```python
from build123d import *

# Parameters (mm, degrees)
STRUCTURAL_MEMBER1_DEPTH = 500
CUT_EXTRUDE1_REACH       = 252.724
LPATTERN1_COUNT          = 196
LPATTERN1_PITCH          = 24.892
SKETCH4_W                = 4000
SKETCH4_H                = 182.847095399
CUT_EXTRUDE2_DEPTH       = 140
SKETCH5_W                = 3.509513676
SKETCH5_H                = 55.564681105
CUT_EXTRUDE3_DEPTH       = 140


with BuildPart() as part:
    # Sketch2 → Structural Member1 (new body)
    with BuildSketch(Plane(origin=(-250, 0, 0), x_dir=(0, 0, -1), z_dir=(1, 0, 0))):
        with BuildLine():
            Line((0, 12.25), (0, -12.25))
            ThreePointArc((0, -12.25), (-0.366116524, -13.133883476), (-1.25, -13.5))
            Line((-1.25, -13.5), (-5.25, -13.5))
            ThreePointArc((-5.25, -13.5), (-6.133883476, -13.866116524), (-6.5, -14.75))
            Line((-6.5, -14.75), (-6.5, -17.5))
            Line((-6.5, -17.5), (-7.5, -17.5))
            Line((-7.5, -17.5), (-7.5, -14.75))
            ThreePointArc((-7.5, -14.75), (-6.840990258, -13.159009742), (-5.25, -12.5))
            Line((-5.25, -12.5), (-1.25, -12.5))
            ThreePointArc((-1.25, -12.5), (-1.073223305, -12.426776695), (-1, -12.25))
            Line((-1, -12.25), (-1, 12.25))
            ThreePointArc((-1, 12.25), (-1.073223305, 12.426776695), (-1.25, 12.5))
            Line((-1.25, 12.5), (-5.25, 12.5))
            ThreePointArc((-5.25, 12.5), (-6.840990258, 13.159009742), (-7.5, 14.75))
            Line((-7.5, 14.75), (-7.5, 17.5))
            Line((-7.5, 17.5), (-6.5, 17.5))
            Line((-6.5, 17.5), (-6.5, 14.75))
            ThreePointArc((-6.5, 14.75), (-6.133883476, 13.866116524), (-5.25, 13.5))
            Line((-5.25, 13.5), (-1.25, 13.5))
            ThreePointArc((-1.25, 13.5), (-0.366116524, 13.133883476), (0, 12.25))
        make_face()
    extrude(amount=STRUCTURAL_MEMBER1_DEPTH)

    # Sketch3 → Cut-Extrude1 (cut, up to next)
    with BuildSketch(Plane.XY, mode=Mode.PRIVATE) as cut_extrude1_sk1:
        with BuildLine():
            Line((-241.745, 3.175), (-230.315, 3.175))
            ThreePointArc((-230.315, 3.175), (-227.14, 0), (-230.315, -3.175))
            Line((-230.315, -3.175), (-241.745, -3.175))
            ThreePointArc((-241.745, -3.175), (-244.92, 0), (-241.745, 3.175))
        make_face()
    cut_extrude1_tool1 = extrude(cut_extrude1_sk1.sketch, amount=CUT_EXTRUDE1_REACH, mode=Mode.PRIVATE) & part.part
    cut_extrude1 = cut_extrude1_tool1.solids().sort_by_distance((-236.03, 0, 0))[0]
    add(cut_extrude1, mode=Mode.SUBTRACT)

    # LPattern1: Cut-Extrude1 ×196
    with Locations(*[(i * LPATTERN1_PITCH, 0, 0) for i in range(1, LPATTERN1_COUNT)]):
        add(cut_extrude1, mode=Mode.SUBTRACT)

    # Sketch4 → Cut-Extrude2 (cut)
    with BuildSketch(Plane.XY.offset(7.5)):
        with Locations((-1947.5, -12.909953422)):
            Rectangle(SKETCH4_W, SKETCH4_H)
    extrude(amount=-CUT_EXTRUDE2_DEPTH, mode=Mode.SUBTRACT)

    # Sketch5 → Cut-Extrude3 (cut)
    with BuildSketch(Plane.XY.offset(7.5)):
        with Locations((249.254756838, -3.17340083)):
            Rectangle(SKETCH5_W, SKETCH5_H)
    extrude(amount=-CUT_EXTRUDE3_DEPTH, mode=Mode.SUBTRACT)


solid = part.part
```
Design review of the part built by this model. Coordinates are the model's own, in mm. A direction names the side the tool comes from. Give positions to 0.01 mm unless a question says otherwise; leave off trailing zeros. Write each loop counter-clockwise with the first axis right and the second up, starting at its lowest first coordinate (ties: lowest second). Pieces come first, ordered by that corner, then holes. Notation, with made-up numbers: (-12, 65.5) - (8, 65.5) arc R21 cw to (8, 73.5) - close; hole circle Ø10 at (60, 58). An arc over 180 degrees is marked (long way). Return JSON: item names as keys, results as strings. Group by question number.
(1) To check wall thickness, follow probe 1 along Y at (x, z) = (193, 5.25); probe 2 along Y at (x, z) = (210.5, 7.25); probe 3 along Z at (x, y) = (178.5, 3.5). State the ranges of each line that lie inside material, in increasing order.
(2) Insertion check: pin 1 (2 mm diameter, centred on x = 129.5, z = 3.5, fed in from -Y); pin 2 (2 mm diameter, centred on x = 185, y = 16.5, fed in from -Z); pin 3 (1.2 mm diameter, centred on x = 152.5, z = 4, fed in from +Y). Each pin has a flat end and moves straight along its axis. Give the tip position at first contact, or say it passes through.
(3) Mouldability with a two-part tool opening along X and no side actions: class faces 5 (the flat face through (149, 0, 0)), 6 (the flat face through (52.5, -0.1, 0.4)), 7 (the cylindrical face through (153.353, -0.07, 0.493)) as +X half, -X half, draft (parallel to the pull), parting line (faces both ways), or undercut.
(4) We need section D-D, the plane y = 10. Give the boundary of the cut face in (x, z), then the cut area to 3 significant figures.
(5) We need section A-A, the plane z = 3.5. Give the boundary of the cut face in (x, y).
(6) We need section C-C, the plane y = 0. Give the number of separate pieces and of enclosed holes in the cut face, then the cut area to 3 significant figures.
(7) Machinability: for faces 1 (the cylindrical face through (196.023, 0.07, 0.493)), 2 (the flat face through (149, -13.5, 3)), 3 (the flat face through (149, -12.5, 3)), 4 (the flat face through (149, 13.5, 3)), which of the approach directions +Z, -Z, +X, -X, +Y, -Y give a long, thin tool a straight path to every point of the face, cutting with its end or side? Answer none if there is none.
(8) We need section B-B, the plane x = 215. Give the boundary of the cut face in (y, z) (3 decimals), then the cut area to 3 significant figures.
Reported:
{
 "1": {"probe 1": "y = -13.5 to -12.5, 12.5 to 13.5", "probe 2": "y = -17.5 to -13.72, 13.72 to 17.5", "probe 3": "z = 0 to 1"},
 "2": {"pin 1": "stops at y = -13.5", "pin 2": "stops at z = 6.5", "pin 3": "stops at y = 13.5"},
 "3": {"face 5": "draft", "face 6": "-X half", "face 7": "undercut"},
 "4": {"outline": "(52.5, 0) - (247.5, 0) - (247.5, 1) - (52.5, 1) - close", "area": "195 mm2"},
 "5": {"outline": "(52.5, -13.5) - (247.5, -13.5) - (247.5, -12.5) - (52.5, -12.5) - close; (52.5, 12.5) - (247.5, 12.5) - (247.5, 13.5) - (52.5, 13.5) - close"},
 "6": {"separate pieces": "9", "enclosed holes": "0", "area": "52.8 mm2"},
 "7": {"face 1": "+Z, -Z", "face 2": "-Z, +X, -X, -Y", "face 3": "+Z, +X, -X", "face 4": "-Z, +X, -X, +Y"},
 "8": {"outline": "(-17.5, 6.5) - (-14.75, 6.5) arc R1.25 cw to (-13.5, 5.25) - (-13.5, 1.25) arc R1.25 ccw to (-12.25, 0) - (-3.175, 0) - (-3.175, 1) - (-12.25, 1) arc R0.25 cw to (-12.5, 1.25) - (-12.5, 5.25) arc R2.25 ccw to (-14.75, 7.5) - (-17.5, 7.5) - close; (3.175, 0) - (12.25, 0) arc R1.25 ccw to (13.5, 1.25) - (13.5, 5.25) arc R1.25 cw to (14.75, 6.5) - (17.5, 6.5) - (17.5, 7.5) - (14.75, 7.5) arc R2.25 ccw to (12.5, 5.25) - (12.5, 1.25) arc R0.25 cw to (12.25, 1) - (3.175, 1) - close", "area": "39.5 mm2"}
}
